Build history of the part. All positions in model axes, mm. Face numbers are marked on the shaded views. Round coordinates to 2 decimals unless told otherwise and drop trailing zeros. Write each loop counter-clockwise with the first axis right and the second up, starting at its lowest first coordinate (ties: lowest second). Pieces come first, ordered by that corner, then holes. Notation, with made-up numbers: M -37,-13 L 14,-13 A30 ccw 14,10 Z; hole C 64.5,8.25 d6. An arc over 180 degrees is marked long. Use a Markdown table: item, result.
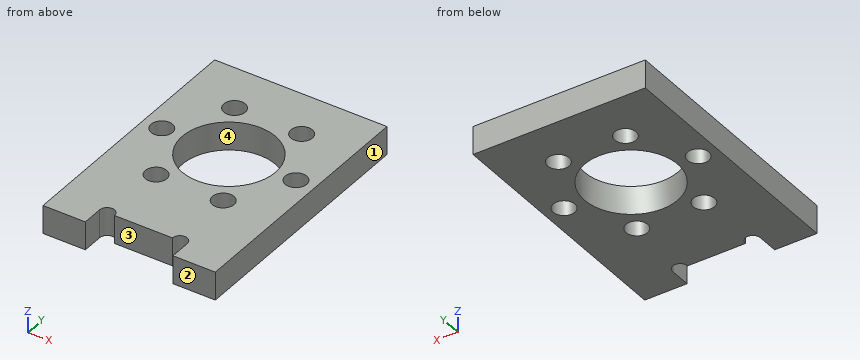
from build123d import *

# Parameters (mm, degrees)
SKETCH_2_W               = 24.4
SKETCH_2_H               = 33
EXTRUDE_1_DEPTH          = 4
SKETCH_3_R               = 6.6
CUT_EXTRUDE_1_DEPTH      = 4
SKETCH_4_W               = 6
SKETCH_4_H               = 3
EXTRUDE_2_DEPTH          = 4
SKETCH_5_R               = 1.05
CUT_EXTRUDE_2_DEPTH      = 4
SKETCH_6_R               = 1.525
CUT_EXTRUDE_3_DEPTH      = 4
PATTERN_CIRCULAR_1_COUNT = 6


with BuildPart() as part:
    # 草图2 → 凸台-拉伸1 (new body)
    with BuildSketch(Plane.XY):
        Rectangle(SKETCH_2_W, SKETCH_2_H)
    extrude(amount=EXTRUDE_1_DEPTH)

    # 草图3 → 切除-拉伸1 (cut)
    with BuildSketch(Plane.XY.offset(4)):
        with Locations((0, 1.410077419)):
            Circle(SKETCH_3_R)
    extrude(amount=-CUT_EXTRUDE_1_DEPTH, mode=Mode.SUBTRACT)

    # 草图4 → 凸台-拉伸2 (add)
    with BuildSketch(Plane.XY.offset(4)):
        with Locations((9.2, -18)):
            Rectangle(SKETCH_4_W, SKETCH_4_H)
    extrude_2 = extrude(amount=-EXTRUDE_2_DEPTH)

    # 镜向1: 凸台-拉伸2 across plane
    add(extrude_2.mirror(Plane(origin=(0, 0, 0), x_dir=(0, 0, 1), z_dir=(1, 0, 0))))

    # 草图5 → 切除-拉伸2 (cut)
    with BuildSketch(Plane(origin=(0, 0, 0), x_dir=(-1, 0, 0), z_dir=(0, 0, -1))):
        with Locations((-5.15, -16.5)):
            Circle(SKETCH_5_R)
        with Locations((5.15, -16.5)):
            Circle(SKETCH_5_R)
    extrude(amount=-CUT_EXTRUDE_2_DEPTH, mode=Mode.SUBTRACT)

    # 草图6 → 切除-拉伸3 (cut)
    with BuildSketch(Plane.XY.offset(4)):
        with Locations((-4.75, -6.817163916)):
            Circle(SKETCH_6_R)
    cut_extrude_3 = extrude(amount=-CUT_EXTRUDE_3_DEPTH, mode=Mode.SUBTRACT)

    # 阵列(圆周)1: 切除-拉伸3 ×6 about axis
    pattern_circular_1_axis = Axis((0, 1.410077419, 0), (0, 0, 1))
    for i in range(1, PATTERN_CIRCULAR_1_COUNT):
        add(cut_extrude_3.rotate(pattern_circular_1_axis, i * 360 / PATTERN_CIRCULAR_1_COUNT), mode=Mode.SUBTRACT)


solid = part.part
Q1. Drop flat-ended pins along their axis: P1, Ø1.8, axis at x = -9.5, y = 1.41, coming from the -Z side; P2, Ø3.5, axis at x = 4.75, y = -6.82, coming from the -Z side; P3, Ø1.2, axis at x = -1.5, z = 2.5, coming from the -Y side. Give the stop position or say it passes through.
Response values:
| item | result |
|---|---|
| P1 | passes through |
| P2 | stops at z = 0 |
| P3 | stops at y = -16.5 |
Q2. Cut at C-C on y = -2. Give the cut face in (x, z), and give its area (3 significant figures).
Response values:
| item | result |
|---|---|
| outline | M -12.2,0 L -5.65,0 L -5.65,4 L -12.2,4 Z; M 5.65,0 L 12.2,0 L 12.2,4 L 5.65,4 Z |
| area | 52.4 mm2 |
Q3. Cut at A-A on x = 9.5. Give the cut face in (y, z), and give its area (3 significant figures).
Response values:
| item | result |
|---|---|
| outline | M -19.5,0 L -0.11,0 L -0.11,4 L -19.5,4 Z; M 2.94,0 L 16.5,0 L 16.5,4 L 2.94,4 Z |
| area | 132 mm2 |
Q4. Two-plate mould, pull along X, no slides. Class the marked faces 1, 2, 3 and 4: +X half, -X half, draft (parallel to the pull), parting line (faces both ways), or undercut.
Response values:
| item | result |
|---|---|
| face 1 | +X half |
| face 2 | draft |
| face 3 | undercut |
| face 4 | undercut |
Q5. Cut at B-B on x = -5.15. Give the cut face in (y, z).
Response values:
| item | result |
|---|---|
| outline | M -15.45,0 L -8.29,0 L -8.29,4 L -15.45,4 Z; M -5.35,0 L -2.72,0 L -2.72,4 L -5.35,4 Z; M 5.54,0 L 8.17,0 L 8.17,4 L 5.54,4 Z; M 11.11,0 L 16.5,0 L 16.5,4 L 11.11,4 Z |
Q6. Cut at D-D on z = 2.4. Count the separate pieces of the cut face and the enclosed holes in it, and give its area (3 significant figures).
Response values:
| item | result |
|---|---|
| separate pieces | 1 |
| enclosed holes | 7 |
| area | 657 mm2 |
Q7. Drill centre lines: L1, parallel to X at y = -18, z = 1.1; L2, parallel to Y at x = 4.5, z = 1.6; L3, parallel to X at y = -6, z = 2.6. Where is each one in solid material? Low to high.
Response values:
| item | result |
|---|---|
| L1 | x = -12.2 to -6.2, 6.2 to 12.2 |
| L2 | y = -15.68 to -8.32, -5.31 to -3.42, 6.24 to 8.13, 11.14 to 16.5 |
| L3 | x = -12.2 to -6.04, -3.46 to 3.46, 6.04 to 12.2 |
